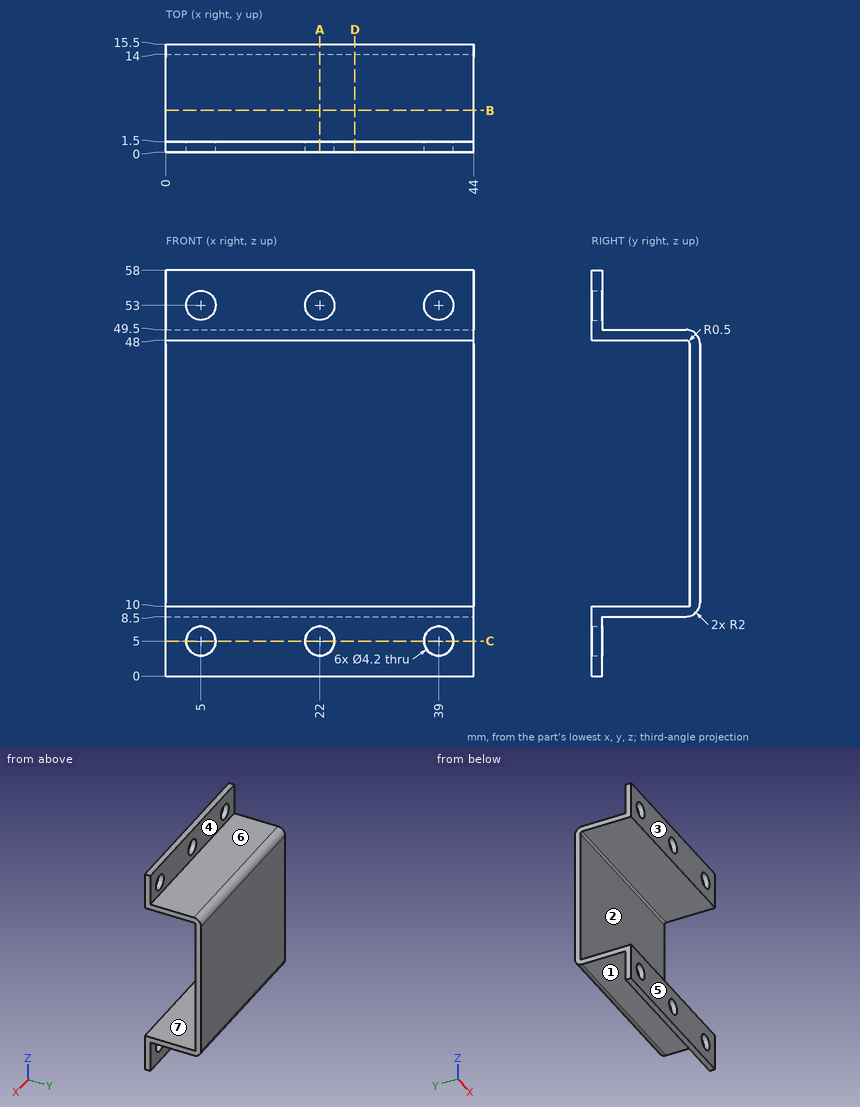
Here's the drawing with two shaded views (mm, measured from the low corner). I have some questions. A direction names the side the tool comes from. Coordinates: 2 decimals unless noted, no trailing zeros. Loops run counter-clockwise (first coordinate to the right, second up) from the corner with the lowest first, then second, coordinate; pieces in that order, holes last. Notation, with made-up numbers: (89.5, 26.5) -> (129.5, 26.5) arc R7 cw to (129.5, 35.5) -> close; hole circle Ø1 at (55, 19.5). An arc over 180 degrees is marked (long way). Put each result on its own line as item: value. Start each with the question number.
Q1. I want a section at D-D (x = 27). Write out the boundary of the cut face in (y, z), plus the area to 3 significant figures.
Q2. If I drill on line 1 (X direction, y = 0.6, z = 53); line 2 (Z direction, x = 5, y = 0.9); line 3 (Z direction, x = 7, y = 1.75), over which ranges is the centre line in solid material (lowest first)? Write a range as [from, to].
Q3. For the marked faces 1, 2, 3 and 4, which set-ups out of +Z, -Z, +X, -X, +Y, -Y let a thin tool reach every point of the face, with its end or its side?
Q4. I want a section at B-B (y = 6). Write out the boundary of the cut face in (x, z).
Q5. I want a section at A-A (x = 22). Write out the boundary of the cut face in (y, z).
Q6. I'm going to push flat-ended pins straight in: P1, Ø6.5, axis at x = 5, z = 53, coming from the -Y side; P2, Ø7, axis at x = 28.5, y = 8, coming from the -Z side; P3, Ø19, axis at x = 17.5, z = 31, coming from the -Y side; P4, Ø3.5, axis at x = 17.5, y = 10, coming from the +Z side. Where does each tip first touch, or does it pass through?
Q7. I want a section at C-C (z = 5). Write out the boundary of the cut face in (x, y).
Q8. Thinking about a two-plate mould opening in Z: for the marked faces 5, 6 and 7, which applies, pulls with the +Z half, pulls with the -Z half, needs draft (parallel to the pull), parting line crosses it, or undercut?
Taken from the geometry:
1. outline: (0, 0) -> (1.5, 0) -> (1.5, 8.5) -> (13.5, 8.5) arc R2 ccw to (15.5, 10.5) -> (15.5, 47.5) arc R2 ccw to (13.5, 49.5) -> (1.5, 49.5) -> (1.5, 58) -> (0, 58) -> (0, 48) -> (13.5, 48) arc R0.5 cw to (14, 47.5) -> (14, 10) -> (0, 10) -> close
1. area: 127 mm2
2. line 1: x = [0, 2.9], [7.1, 19.9], [24.1, 36.9], [41.1, 44]
2. line 2: z = [0, 2.9], [7.1, 10], [48, 50.9], [55.1, 58]
2. line 3: z = [8.5, 10], [48, 49.5]
3. face 1: -Z, +X, -X, +Y
3. face 2: +X, -X, -Y
3. face 3: +Z, -Z, +X, -X, -Y
3. face 4: +Z, +X, -X, +Y
4. outline: (0, 8.5) -> (44, 8.5) -> (44, 10) -> (0, 10) -> close; (0, 48) -> (44, 48) -> (44, 49.5) -> (0, 49.5) -> close
5. outline: (0, 0) -> (1.5, 0) -> (1.5, 2.9) -> (0, 2.9) -> close; (0, 7.1) -> (1.5, 7.1) -> (1.5, 8.5) -> (13.5, 8.5) arc R2 ccw to (15.5, 10.5) -> (15.5, 47.5) arc R2 ccw to (13.5, 49.5) -> (1.5, 49.5) -> (1.5, 50.9) -> (0, 50.9) -> (0, 48) -> (13.5, 48) arc R0.5 cw to (14, 47.5) -> (14, 10) -> (0, 10) -> close; (0, 55.1) -> (1.5, 55.1) -> (1.5, 58) -> (0, 58) -> close
6. P1: stops at y = 0
6. P2: stops at z = 8.5
6. P3: stops at y = 14
6. P4: stops at z = 49.5
7. outline: (0, 0) -> (2.9, 0) -> (2.9, 1.5) -> (0, 1.5) -> close; (7.1, 0) -> (19.9, 0) -> (19.9, 1.5) -> (7.1, 1.5) -> close; (24.1, 0) -> (36.9, 0) -> (36.9, 1.5) -> (24.1, 1.5) -> close; (41.1, 0) -> (44, 0) -> (44, 1.5) -> (41.1, 1.5) -> close
8. face 5: needs draft
8. face 6: pulls with the +Z half
8. face 7: undercut
